Read the model definition and answer for the solid it produces. Units are mm, in the model's axes. Coordinates: 2 decimals unless noted, no trailing zeros. Loops run counter-clockwise (first coordinate to the right, second up) from the corner with the lowest first, then second, coordinate; pieces in that order, holes last.
from build123d import *

# Parameters (mm, degrees)
PANEL_W             = 403
PANEL_H             = 78
BOSS_EXTRUDE1_DEPTH = 1.6
ROCKER_SWITCH_W     = 12.9
ROCKER_SWITCH_H     = 19.33
CUT_EXTRUDE2_DEPTH  = 10
CUT_EXTRUDE4_DEPTH  = 10
CUT_EXTRUDE6_DEPTH  = 10


with BuildPart() as part:
    # Panel → Boss-Extrude1 (new body)
    with BuildSketch(Plane.XY):
        with Locations((201.5, 39)):
            Rectangle(PANEL_W, PANEL_H)
    extrude(amount=BOSS_EXTRUDE1_DEPTH)

    # Rocker_Switch → Cut-Extrude2 (cut)
    with BuildSketch(Plane.XY.offset(1.6)):
        with Locations((56.45, 44.665)):
            Rectangle(ROCKER_SWITCH_W, ROCKER_SWITCH_H)
    extrude(amount=-CUT_EXTRUDE2_DEPTH, mode=Mode.SUBTRACT)

    # Turbo → Cut-Extrude4 (cut)
    with BuildSketch(Plane.XY):
        with BuildLine():
            Line((197.216263462, 52.500054059), (202.783736538, 52.500054059))
            ThreePointArc((202.783736538, 52.500054059), (208, 45), (202.783736538, 37.499945941))
            Line((202.783736538, 37.499945941), (197.216263462, 37.499945941))
            ThreePointArc((197.216263462, 37.499945941), (192, 45), (197.216263462, 52.500054059))
        make_face()
    extrude(amount=CUT_EXTRUDE4_DEPTH, mode=Mode.SUBTRACT)

    # En/Disable → Cut-Extrude6 (cut)
    with BuildSketch(Plane.XY.offset(1.6)):
        with BuildLine():
            Line((127.216263462, 52.500054059), (132.783736538, 52.500054059))
            ThreePointArc((132.783736538, 52.500054059), (138, 45), (132.783736538, 37.499945941))
            Line((132.783736538, 37.499945941), (127.216263462, 37.499945941))
            ThreePointArc((127.216263462, 37.499945941), (122, 45), (127.216263462, 52.500054059))
        make_face()
    extrude(amount=-CUT_EXTRUDE6_DEPTH, mode=Mode.SUBTRACT)


solid = part.part
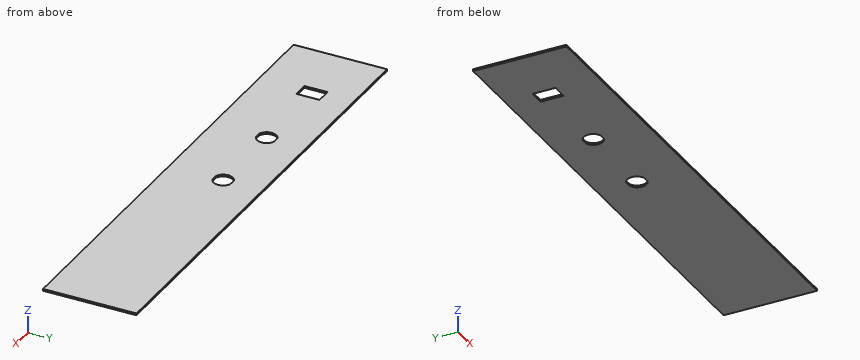
Item 1: A cutting plane is placed at A-A on z = 0.4. Determine the outline of the cut face in (x, y), then the cut area to 3 significant figures.
Numbers:
outline: (0, 0) - (403, 0) - (403, 78) - (0, 78) - close; hole (50, 35) - (62.9, 35) - (62.9, 54.33) - (50, 54.33) - close; hole (127.22, 37.5) - (132.78, 37.5) arc R8 ccw to (132.78, 52.5) - (127.22, 52.5) arc R8 ccw to start; hole (197.22, 37.5) - (202.78, 37.5) arc R8 ccw to (202.78, 52.5) - (197.22, 52.5) arc R8 ccw to start
area: 30,800 mm2
Item 2: A cutting plane is placed at B-B on y = 47.5. Determine the outline of the cut face in (x, z).
Numbers:
outline: (0, 0) - (50, 0) - (50, 1.6) - (0, 1.6) - close; (62.9, 0) - (122.4, 0) - (122.4, 1.6) - (62.9, 1.6) - close; (137.6, 0) - (192.4, 0) - (192.4, 1.6) - (137.6, 1.6) - close; (207.6, 0) - (403, 0) - (403, 1.6) - (207.6, 1.6) - close
Item 3: Find the intervals of material crossed by line 1 along X through (y, z) = (44, 1.1); line 2 along X through (y, z) = (37, 0.1); line 3 along X through (y, z) = (41, 0.3), in increasing order.
Numbers:
line 1: x = 0 to 50, 62.9 to 122.06, 137.94 to 192.06, 207.94 to 403
line 2: x = 0 to 50, 62.9 to 403
line 3: x = 0 to 50, 62.9 to 123.07, 136.93 to 193.07, 206.93 to 403
